The figure shows three views and two pictorial views of one solid part (mm, origin at its lowest corner). Answer the questions. Give positions to 0.01 mm unless a question says otherwise; leave off trailing zeros. Answer as CSV lines item,"result". Start each with the question number.
1. Section B-B on x = 139.7 is taken. Count the separate pieces of the cut face and the enclosed holes in it, and give its area (3 significant figures).
2. Flat-ended cylindrical pins translate along their axes: pin 1 (2.5 mm diameter, centred on x = 63.5, z = 25.4, fed in from +Y) (1 decimal); pin 2 (5 mm diameter, centred on x = 63.5, z = 12.7, fed in from -Y); pin 3 (1.9 mm diameter, centred on x = 142, y = 2, fed in from -Z) (3 decimals). Find the tip coordinate at first contact, or state that the pin passes through.
3. Consider line 1 along Z through (x, y) = (88.9, 4.5) (1 decimal); line 2 along Z through (x, y) = (12.7, 2) (1 decimal); line 3 along X through (y, z) = (2.25, 50.8) (1 decimal). Determine where each line is inside the solid, lowest interval first. Write a range as [from, to].
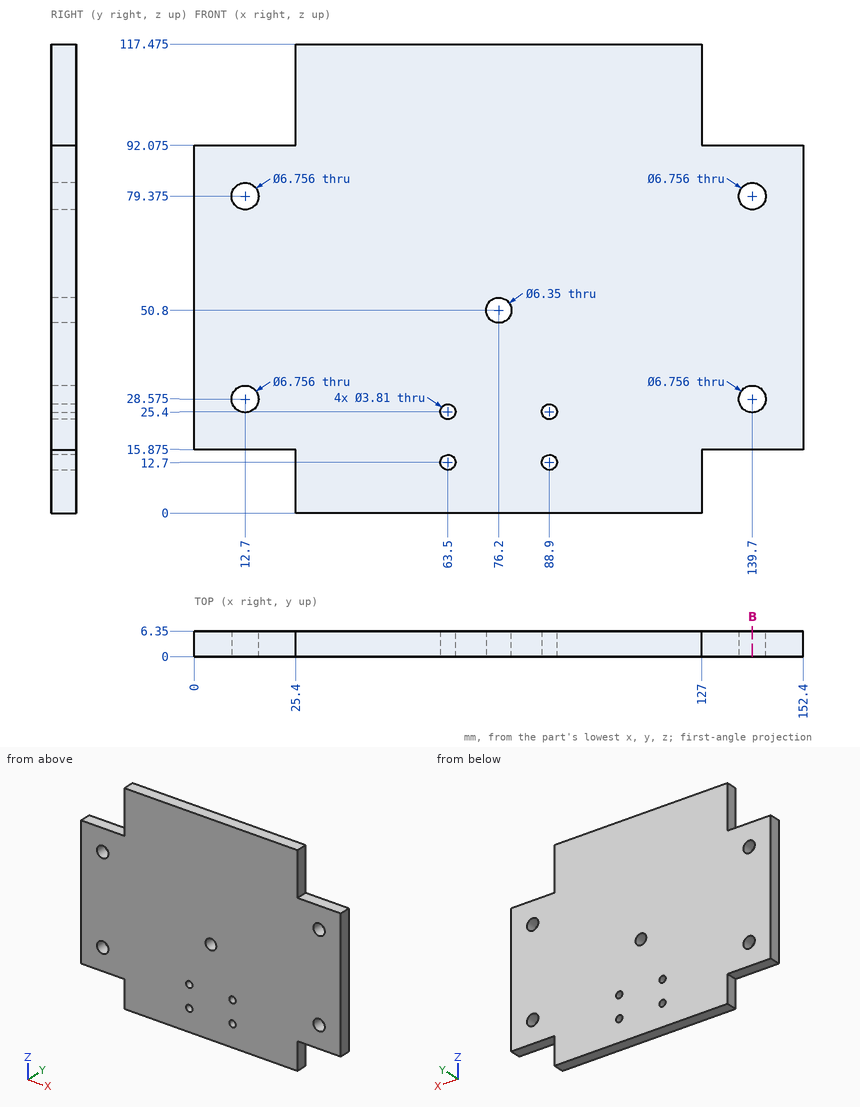
Checks:
1,separate pieces,"3"
1,enclosed holes,"0"
1,area,"398 mm²"
2,pin 1,"passes through"
2,pin 2,"stops at y = 0"
2,pin 3,"stops at z = 15.875"
3,line 1,"z = [0, 10.8], [14.6, 23.5], [27.3, 117.5]"
3,line 2,"z = [15.9, 25.2], [32, 76], [82.8, 92.1]"
3,line 3,"x = [0, 73], [79.4, 152.4]"
